Input: part model. Units: mm. Frame: model coordinates. Give positions to 0.01 mm unless a question says otherwise; leave off trailing zeros. Loops run counter-clockwise (first coordinate to the right, second up) from the corner with the lowest first, then second, coordinate; pieces in that order, holes last. Notation, with made-up numbers: M 12,58 L 33,58 A32 cw 33,92 Z; hole C -23.75,64 d8. An arc over 180 degrees is marked long. Use CSV: the item, a comma, the result in double quotes. Start each with the question number.
Q1. Section A-A, the plane x = 11. Output: boundary loops of the cut face in (y, z) (1 decimal), plus the area to 3 significant figures.
Q2. Section B-B, the plane z = 25. Output: boundary loops of the cut face in (x, y) (3 decimals), plus the area to 3 significant figures.
Q3. Material intervals for line 1 along Z through (x, y) = (-20, 1) (1 decimal); line 2 along X through (y, z) = (1.95, 0) (3 decimals); line 3 along X through (y, z) = (0.5, -28.5) (3 decimals), sorted ascending.
Q4. Section C-C, the plane x = 78. Output: boundary loops of the cut face in (y, z) (3 decimals).
Q5. Pin query (flat end, axial travel): pin 1 (1 mm diameter, centred on x = 32.5, z = -21, fed in from -Y); pin 2 (1 mm diameter, centred on y = 2, z = -26, fed in from -X) (3 decimals); pin 3 (1 mm diameter, centred on x = -73.5, y = 2.5, fed in from -Z) (3 decimals); pin 4 (1.6 mm diameter, centred on y = 1, z = 37, fed in from -X). Return the tip coordinate at first contact, or that it passes through.
from build123d import *

# Parameters (mm, degrees)
SKETCH1_W           = 203.2
SKETCH1_H           = 76.2
BOSS_EXTRUDE1_DEPTH = 3.175
SKETCH2_W           = 40.64
SKETCH2_H           = 3.175
CUT_EXTRUDE1_DEPTH  = 3.175
LPATTERN1_COUNT     = 3
LPATTERN1_PITCH     = 81.28
SKETCH3_W           = 3.175
SKETCH3_H           = 15.24
CUT_EXTRUDE2_DEPTH  = 3.175
LPATTERN2_COUNT     = 3
LPATTERN2_PITCH     = 30.48
SKETCH4_W           = 40.64
SKETCH4_H           = 3.175
CUT_EXTRUDE3_DEPTH  = 3.175


with BuildPart() as part:
    # Sketch1 → Boss-Extrude1 (new body)
    with BuildSketch(Plane(origin=(0, 0, 0), x_dir=(1, 0, 0), z_dir=(0, 1, 0))):
        Rectangle(SKETCH1_W, SKETCH1_H)
    extrude(amount=BOSS_EXTRUDE1_DEPTH)

    # Sketch2 → Cut-Extrude1 (cut)
    with BuildSketch(Plane(origin=(0, 3.175, 0), x_dir=(1, 0, 0), z_dir=(0, 1, 0))):
        with Locations((-81.28, 36.5125)):
            Rectangle(SKETCH2_W, SKETCH2_H)
        with Locations((-81.28, -36.5125)):
            Rectangle(SKETCH2_W, SKETCH2_H)
    cut_extrude1 = extrude(amount=-CUT_EXTRUDE1_DEPTH, mode=Mode.SUBTRACT)

    # LPattern1: Cut-Extrude1 ×3
    with Locations(*[(i * LPATTERN1_PITCH, 0, 0) for i in range(1, LPATTERN1_COUNT)]):
        add(cut_extrude1, mode=Mode.SUBTRACT)

    # Sketch3 → Cut-Extrude2 (cut)
    with BuildSketch(Plane(origin=(0, 3.175, 0), x_dir=(1, 0, 0), z_dir=(0, 1, 0))):
        with Locations((100.0125, 30.48)):
            Rectangle(SKETCH3_W, SKETCH3_H)
        with Locations((-100.0125, 30.48)):
            Rectangle(SKETCH3_W, SKETCH3_H)
    cut_extrude2 = extrude(amount=-CUT_EXTRUDE2_DEPTH, mode=Mode.SUBTRACT)

    # LPattern2: Cut-Extrude2 ×3
    with Locations(*[(0, 0, i * LPATTERN2_PITCH) for i in range(1, LPATTERN2_COUNT)]):
        add(cut_extrude2, mode=Mode.SUBTRACT)

    # Sketch4 → Cut-Extrude3 (cut)
    with BuildSketch(Plane(origin=(0, 3.175, 0), x_dir=(1, 0, 0), z_dir=(0, 1, 0))):
        Rectangle(SKETCH4_W, SKETCH4_H)
    extrude(amount=-CUT_EXTRUDE3_DEPTH, mode=Mode.SUBTRACT)


solid = part.part
A:
1,outline,"M 0,-34.9 L 3.2,-34.9 L 3.2,-1.6 L 0,-1.6 Z; M 0,1.6 L 3.2,1.6 L 3.2,34.9 L 0,34.9 Z"
1,area,"212 mm^2"
2,outline,"M -98.425,0 L 98.425,0 L 98.425,3.175 L -98.425,3.175 Z"
2,area,"625 mm^2"
3,line 1,"-34.9 to -1.6, 1.6 to 34.9"
3,line 2,"-98.425 to -20.32, 20.32 to 98.425"
3,line 3,"-98.425 to 98.425"
4,outline,"M 0,-34.925 L 3.175,-34.925 L 3.175,34.925 L 0,34.925 Z"
5,pin 1,"y = 0"
5,pin 2,"x = -98.425"
5,pin 3,"z = -34.925"
5,pin 4,"x = -60.96"
